Could you check a few things on this drawing? It's one solid part, dimensions in mm from its lowest x, y, z. A direction names the side the tool comes from. Coordinates: 2 decimals unless noted, no trailing zeros. Order: outer loops, then holes, each group sorted by start corner. A loop starts at its lowest first (then second) coordinate and runs counter-clockwise, first axis right, second up.
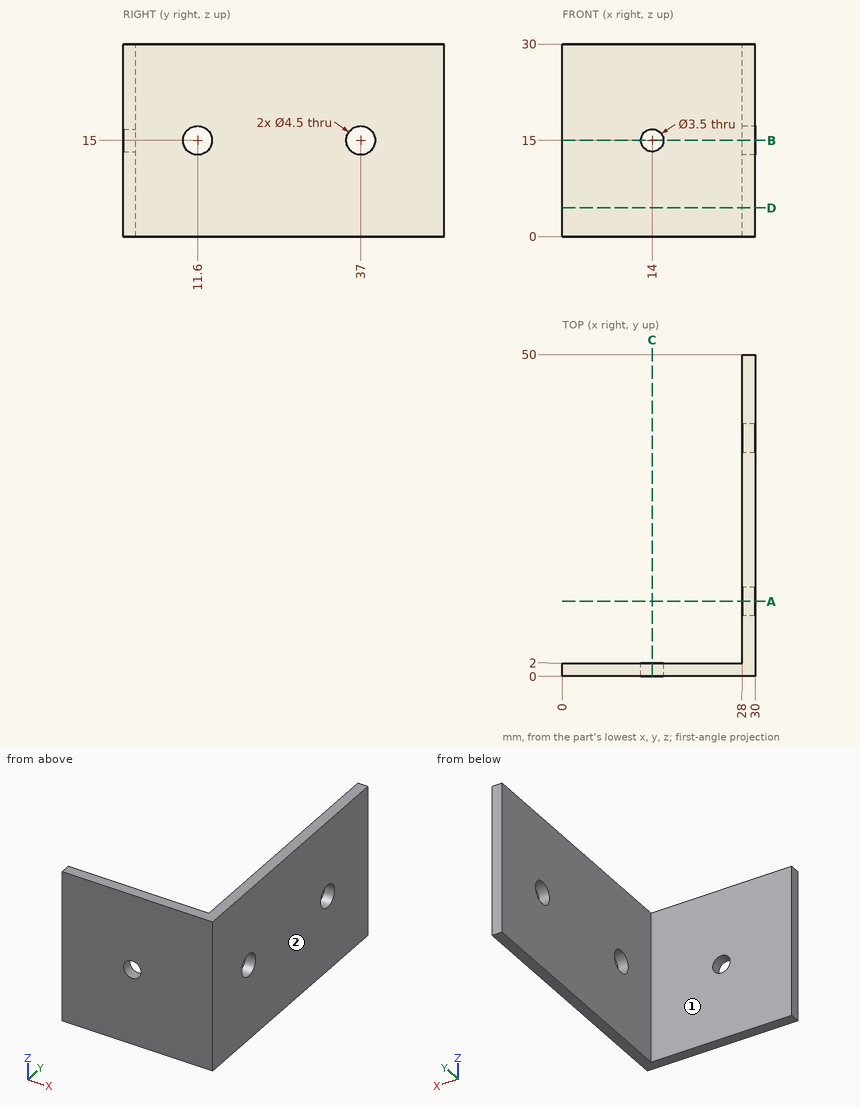
Q1. If we section it at A-A on y = 11.6: Write out the boundary of the cut face in (x, z), then the cut area to 3 significant figures.
Q2. If we section it at C-C on x = 14: Write out the boundary of the cut face in (y, z), then the cut area to 3 significant figures.
Q3. If we section it at D-D on z = 4.5: Write out the boundary of the cut face in (x, y).
Q4. If we section it at B-B on z = 15: Write out the boundary of the cut face in (x, y).
Q5. For the marked faces 1 and 2, which set-ups out of +Z, -Z, +X, -X, +Y, -Y let a thin tool reach every point of the face, with its end or its side?
Q6. Will these pins go through, and if not, where does the flat tip stop? pin 1 (6 mm diameter, centred on x = 24, z = 21, fed in from +Y); pin 2 (3 mm diameter, centred on y = 40, z = 23.5, fed in from -X).
Q7. I need wall thicknesses on L1, parallel to Y at x = 29.55, z = 15; L2, parallel to Z at x = 14, y = 0.7; L3, parallel to X at y = 0.95, z = 15. Which ranges of each line are inside material? Lowest first, please.
Reply:
1. outline: (28, 0) - (30, 0) - (30, 12.75) - (28, 12.75) - close; (28, 17.25) - (30, 17.25) - (30, 30) - (28, 30) - close
1. area: 51.0 mm2
2. outline: (0, 0) - (2, 0) - (2, 13.25) - (0, 13.25) - close; (0, 16.75) - (2, 16.75) - (2, 30) - (0, 30) - close
2. area: 53.0 mm2
3. outline: (0, 0) - (30, 0) - (30, 50) - (28, 50) - (28, 2) - (0, 2) - close
4. outline: (0, 0) - (12.25, 0) - (12.25, 2) - (0, 2) - close; (15.75, 0) - (30, 0) - (30, 9.35) - (28, 9.35) - (28, 2) - (15.75, 2) - close; (28, 13.85) - (30, 13.85) - (30, 34.75) - (28, 34.75) - close; (28, 39.25) - (30, 39.25) - (30, 50) - (28, 50) - close
5. face 1: +Z, -Z, -X, +Y
5. face 2: +Z, -Z, +X, +Y, -Y
6. pin 1: stops at y = 2
6. pin 2: stops at x = 28
7. L1: y = 0 to 9.35, 13.85 to 34.75, 39.25 to 50
7. L2: z = 0 to 13.25, 16.75 to 30
7. L3: x = 0 to 12.25, 15.75 to 30
